Read the model definition and answer for the solid it produces. Units are mm, in the model's axes. Give positions to 0.01 mm unless a question says otherwise; leave off trailing zeros. Order: outer loops, then holes, each group sorted by start corner. A loop starts at its lowest first (then second) coordinate and runs counter-clockwise, first axis right, second up. Notation, with made-up numbers: (-0.5, 17) -> (20.5, 17) arc R20 ccw to (20.5, 35) -> close; hole circle Ø2 at (58.5, 39.25). An arc over 180 degrees is marked (long way). One line per item, written item: value. Start each with the question number.
from build123d import *

# Parameters (mm, degrees)
SKETCH1_W           = 100
SKETCH1_H           = 60
BOSS_EXTRUDE1_DEPTH = 30
BOSS_EXTRUDE2_DEPTH = 100
SKETCH4_R           = 7.5
CUT_EXTRUDE1_DEPTH  = 100


with BuildPart() as part:
    # Sketch1 → Boss-Extrude1 (new body)
    with BuildSketch(Plane(origin=(0, 0, 0), x_dir=(1, 0, 0), z_dir=(0, 1, 0))):
        Rectangle(SKETCH1_W, SKETCH1_H)
    extrude(amount=BOSS_EXTRUDE1_DEPTH)

    # Sketch2 → Boss-Extrude2 (add)
    with BuildSketch(Plane(origin=(50, 0, 0), x_dir=(0, 0, -1), z_dir=(1, 0, 0))):
        with BuildLine():
            Line((-30, 30), (30, 30))
            add(Edge.make_bspline(
                [(30, 30), (15.504637598, 46.413049946), (14.954961798, 65.984799867)],
                knots=[0, 0, 0, 1, 1, 1], degree=2))
            ThreePointArc((14.954961798, 65.984799867), (0.029992259, 79.823254651), (-14.950197367, 66.044594871))
            add(Edge.make_bspline(
                [(-30, 30), (-15.530658632, 46.442080305), (-14.950197367, 66.044594871)],
                knots=[0, 0, 0, 1, 1, 1], degree=2))
        make_face()
    extrude(amount=-BOSS_EXTRUDE2_DEPTH)

    # Sketch4 → Cut-Extrude1 (cut)
    with BuildSketch(Plane(origin=(50, 0, 0), x_dir=(0, 0, -1), z_dir=(1, 0, 0))):
        with Locations((0, 64.823284635)):
            Circle(SKETCH4_R)
        with Locations((-15, 15.336875133)):
            Circle(SKETCH4_R)
        with Locations((15, 15.336875133)):
            Circle(SKETCH4_R)
    extrude(amount=-CUT_EXTRUDE1_DEPTH, mode=Mode.SUBTRACT)


solid = part.part
Item 1: Find section B-B on y = 71. Write down the section's boundary in (x, z).
Item 2: Find section C-C on y = 13. Write down the section's boundary in (x, z), then the cut area to 3 significant figures.
Item 3: Find section A-A on z = 0. Write down the section's boundary in (x, y).
Item 4: For a pull along Z with two mould halves and no side action, classify faces 1 (the flat face through (-1, 15, 30)), 2 (the flat face through (50, 32, 0)), 3 (the cylindrical face through (0.7, 8.015, -13.374)) as +Z half, -Z half, draft (parallel to the pull), parting line (faces both ways), or undercut.
Item 5: Find the intervals of material crossed by line 1 (Z direction, x = 7.5, y = 9); line 2 (Y direction, x = 12, z = 0); line 3 (Z direction, x = -21, y = 64.5), in increasing order. Write a range as from..to.
Item 6: Flat-ended cylindrical pins translate along their axes: pin 1 (6 mm diameter, centred on y = 11.5, z = -18.5, fed in from -X); pin 2 (6 mm diameter, centred on x = -19, z = -10.5, fed in from +Y); pin 3 (6 mm diameter, centred on x = 14, y = 57, fed in from -Z). Find the tip coordinate at first contact, or state that the pin passes through.
Item 7: Find section D-D on x = -0.5. Count the separate pieces of the cut face and the enclosed holes in it, then the cut area to 3 significant figures.
Checks:
1. outline: (-50, -13.67) -> (50, -13.67) -> (50, -4.25) -> (-50, -4.25) -> close; (-50, 4.25) -> (50, 4.25) -> (50, 13.67) -> (-50, 13.67) -> close
2. outline: (-50, -30) -> (50, -30) -> (50, -22.13) -> (-50, -22.13) -> close; (-50, -7.87) -> (50, -7.87) -> (50, 7.87) -> (-50, 7.87) -> close; (-50, 22.13) -> (50, 22.13) -> (50, 30) -> (-50, 30) -> close
2. area: 3,150 mm2
3. outline: (-50, 0) -> (50, 0) -> (50, 57.32) -> (-50, 57.32) -> close; (-50, 72.32) -> (50, 72.32) -> (50, 79.82) -> (-50, 79.82) -> close
4. face 1: +Z half
4. face 2: draft
4. face 3: undercut
5. line 1: -30..-19.01, -10.99..10.99, 19.01..30
5. line 2: 0..57.32, 72.32..79.82
5. line 3: -15.02..-7.49, 7.49..15.02
6. pin 1: x = -50
6. pin 2: y = 77.81
6. pin 3: z = -16.68
7. separate pieces: 1
7. enclosed holes: 3
7. area: 3,020 mm2
